Geometry: final body of the model. Coordinates: model frame, mm. Face numbers are marked on the shaded views. A direction names the side the tool comes from. Coordinates: 2 decimals unless noted, no trailing zeros. Loops run counter-clockwise (first coordinate to the right, second up) from the corner with the lowest first, then second, coordinate; pieces in that order, holes last. Notation, with made-up numbers: (52.5, 25.25) - (84.5, 25.25) arc R7 cw to (84.5, 31.25) - close; hole circle Ø4 at (5.5, 84). An arc over 180 degrees is marked (long way). Put each result on its own line as item: value. Start each with the question number.
1) Section A-A on x = 23.35. Output: boundary loops of the cut face in (y, z).
2) Contact query for flat-ended pins moving along their axis: pin 1 Ø4 at (x, z) = (37, -5) entering from -Y; pin 2 Ø1.5 at (x, y) = (27.5, 7) entering from +Z; pin 3 Ø1.5 at (x, z) = (-40.5, 27) entering from +Y; pin 4 Ø2 at (x, z) = (-42.5, 15.5) entering from +Y. Output: stop coordinate, or through.
3) Section D-D on x = 8. Output: boundary loops of the cut face in (y, z).
4) Section B-B on z = 27. Output: boundary loops of the cut face in (x, y), and give its area (3 significant figures).
5) Material intervals for line 1 along X through (y, z) = (4.75, -30.5); line 2 along X through (y, z) = (6.5, -26.5); line 3 along X through (y, z) = (7, -12.25), sorted ascending. Write a range as from..to.
6) Reachability of the marked faces 1 and 2 from +Z, -Z, +X, -X, +Y, -Y: full face, straight path, thin tool, end or side. Return the list, or none.
7) Section C-C on x = -23.5. Output: boundary loops of the cut face in (y, z), and give its area (3 significant figures).
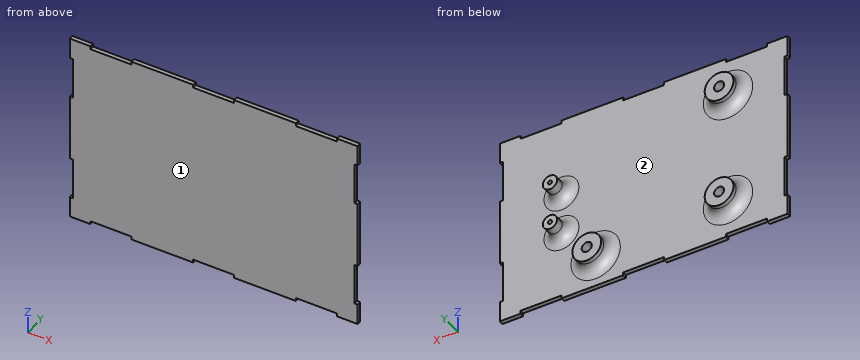
```python
from build123d import *

# Parameters (mm, degrees)
SKETCH1_W           = 140
SKETCH1_H           = 92
BOSS_EXTRUDE1_DEPTH = 2.1
SKETCH2_W           = 1.5
SKETCH2_H           = 20
SKETCH2_W_2         = 20
SKETCH2_H_2         = 1.5
CUT_EXTRUDE1_DEPTH  = 84.787886953
SKETCH3_R           = 7
SKETCH3_R_2         = 3.5
BOSS_EXTRUDE2_DEPTH = 7
SKETCH6_R           = 3.5
BOSS_EXTRUDE3_DEPTH = 2
SKETCH7_R           = 2.45
CUT_EXTRUDE4_DEPTH  = 5.1
SKETCH8_R           = 1
CUT_EXTRUDE5_DEPTH  = 7
FILLET1_R           = 5


with BuildPart() as part:
    # Sketch1 → Boss-Extrude1 (new body)
    with BuildSketch(Plane(origin=(0, 0, 0), x_dir=(1, 0, 0), z_dir=(0, 1, 0))):
        Rectangle(SKETCH1_W, SKETCH1_H)
    extrude(amount=BOSS_EXTRUDE1_DEPTH)

    # Sketch2 → Cut-Extrude1 (cut, through all)
    with BuildSketch(Plane(origin=(0, 2.1, 0), x_dir=(1, 0, 0), z_dir=(0, 1, 0))):
        with Locations((69.25, 26)):
            Rectangle(SKETCH2_W, SKETCH2_H)
        with Locations((69.25, -26)):
            Rectangle(SKETCH2_W, SKETCH2_H)
        with Locations((50, -45.25)):
            Rectangle(SKETCH2_W_2, SKETCH2_H_2)
        with Locations((-50, -45.25)):
            Rectangle(SKETCH2_W_2, SKETCH2_H_2)
        with Locations((0, -45.25)):
            Rectangle(SKETCH2_W_2, SKETCH2_H_2)
        with Locations((-50, 45.25)):
            Rectangle(SKETCH2_W_2, SKETCH2_H_2)
        with Locations((0, 45.25)):
            Rectangle(SKETCH2_W_2, SKETCH2_H_2)
        with Locations((50, 45.25)):
            Rectangle(SKETCH2_W_2, SKETCH2_H_2)
        with Locations((-69.25, 26)):
            Rectangle(SKETCH2_W, SKETCH2_H)
        with Locations((-69.25, -26)):
            Rectangle(SKETCH2_W, SKETCH2_H)
    extrude(amount=-CUT_EXTRUDE1_DEPTH, mode=Mode.SUBTRACT)

    # Sketch3 → Boss-Extrude2 (add)
    with BuildSketch(Plane(origin=(0, 2.1, 0), x_dir=(1, 0, 0), z_dir=(0, 1, 0))):
        with Locations(Location((-41.05, 27.5, 0), (0, 0, 90))):
            Circle(SKETCH3_R)
        with Locations(Location((-41.05, -27, 0), (0, 0, 90))):
            Circle(SKETCH3_R)
        with Locations(Location((23.35, 30.5, 0), (0, 0, 90))):
            Circle(SKETCH3_R)
        with Locations(Location((40, 12.25, 0), (0, 0, 90))):
            Circle(SKETCH3_R_2)
        with Locations(Location((40, -8.25, 0), (0, 0, 90))):
            Circle(SKETCH3_R_2)
    extrude(amount=BOSS_EXTRUDE2_DEPTH)

    # Sketch6 → Boss-Extrude3 (add)
    with BuildSketch(Plane(origin=(0, 9.1, 0), x_dir=(1, 0, 0), z_dir=(0, 1, 0))):
        with Locations(Location((40, 12.25, 0), (0, 0, 90))):
            Circle(SKETCH6_R)
        with Locations(Location((40, -8.25, 0), (0, 0, 90))):
            Circle(SKETCH6_R)
    extrude(amount=BOSS_EXTRUDE3_DEPTH)

    # Sketch7 → Cut-Extrude4 (cut)
    with BuildSketch(Plane(origin=(0, 9.1, 0), x_dir=(1, 0, 0), z_dir=(0, 1, 0))):
        with Locations(Location((-41.05, 27.5, 0), (0, 0, 270))):
            Circle(SKETCH7_R)
        with Locations(Location((23.35, 30.5, 0), (0, 0, 270))):
            Circle(SKETCH7_R)
        with Locations(Location((-41.05, -27, 0), (0, 0, 270))):
            Circle(SKETCH7_R)
    extrude(amount=-CUT_EXTRUDE4_DEPTH, mode=Mode.SUBTRACT)

    # Sketch8 → Cut-Extrude5 (cut)
    with BuildSketch(Plane(origin=(0, 11.1, 0), x_dir=(1, 0, 0), z_dir=(0, 1, 0))):
        with Locations(Location((40, 12.25, 0), (0, 0, 270))):
            Circle(SKETCH8_R)
        with Locations(Location((40, -8.25, 0), (0, 0, 270))):
            Circle(SKETCH8_R)
    extrude(amount=-CUT_EXTRUDE5_DEPTH, mode=Mode.SUBTRACT)

    # Fillet1
    fillet1_edges = [part.edges().sort_by_distance(p)[0] for p in [
        (-41.05, 2.1, -20.5),
        (-41.05, 2.1, 34),
        (23.35, 2.1, -23.5),
        (40, 2.1, -8.75),
        (40, 2.1, 11.75),
    ]]
    fillet(fillet1_edges, radius=FILLET1_R)


solid = part.part
```
Answer block:
1. outline: (0, -46) - (2.1, -46) - (2.1, -42.5) arc R5 cw to (7.1, -37.5) - (9.1, -37.5) - (9.1, -32.95) - (4, -32.95) - (4, -28.05) - (9.1, -28.05) - (9.1, -23.5) - (7.1, -23.5) arc R5 cw to (2.1, -18.5) - (2.1, 46) - (0, 46) - close
2. pin 1: stops at y = 0
2. pin 2: stops at z = -24.38
2. pin 3: stops at y = 4
2. pin 4: stops at y = 2.3
3. outline: (0, -44.5) - (2.1, -44.5) - (2.1, 44.5) - (0, 44.5) - close
4. outline: (-68.5, 0) - (68.5, 0) - (68.5, 2.1) - (-29.05, 2.1) arc R5 cw to (-34.05, 7.1) - (-34.05, 9.1) - (-38.6, 9.1) - (-38.6, 4) - (-43.5, 4) - (-43.5, 9.1) - (-48.05, 9.1) - (-48.05, 7.1) arc R5 cw to (-53.05, 2.1) - (-68.5, 2.1) - close
4. area: 371 mm²
5. line 1: x = -48.02..-34.08, 15.76..20.9, 25.8..30.94
5. line 2: x = -48.01..-43.29, -38.81..-34.09, 17.56..29.14
5. line 3: x = 36.5..39, 41..43.5
6. face 1: +Z, -Z, +X, -X, -Y
6. face 2: +Y
7. outline: (0, -46) - (2.1, -46) - (2.1, 46) - (0, 46) - close
7. area: 193 mm²
